Here's how the part is built. I have some questions about the finished solid (model axes, mm). A direction names the side the tool comes from. Round coordinates to 2 decimals unless told otherwise and drop trailing zeros. Write each loop counter-clockwise with the first axis right and the second up, starting at its lowest first coordinate (ties: lowest second). Pieces come first, ordered by that corner, then holes. Notation, with made-up numbers: M 89,-25.5 L 148,-25.5 A22 cw 148,-4.5 Z; hole C 79,63.25 d2. An arc over 180 degrees is marked long. Use one line per item in the form item = value. Start each with the question number.
Q1. I need wall thicknesses on line 1 along Y through (x, z) = (0, 16); line 2 along Y through (x, z) = (0, 3); line 3 along Z through (x, y) = (-8, 13). Which ranges of each line are inside material? Lowest first, please. Write a range as from..to.
Q2. I want a section at D-D on x = -18.5. List the corners of the cut face in (y, z) for me.
Q3. I want a section at C-C on y = 30. List the corners of the cut face in (x, z) for me.
Q4. I want a section at A-A on z = 4. List the corners of the cut face in (x, y) for me.
Q5. I want a section at B-B on x = 4. List the corners of the cut face in (y, z) for me.
Q6. We'd pull the mould along X, two halves only. Please class faces 1 (the face through (28, 0, 60)), 2 (the face through (24.5, 2.65, 55.08)), 3 (the face through (-20.23, 3.62, 9.86)): +X half, -X half, draft (parallel to the pull), parting line (faces both ways), or undercut.
Q7. I'm going to push flat-ended pins straight in: pin 1 Ø13.5 at (x, y) = (2.5, 14.5) entering from +Z; pin 2 Ø5 at (x, y) = (28.5, 8.5) entering from +Z; pin 3 Ø2 at (y, z) = (-1, 15) entering from +X; pin 4 Ø8 at (y, z) = (5.5, 45.5) entering from -X. Where does each tip first touch, or does it pass through?
Q8. For faces 4 (the face through (24.43, -0.61, 44.08)), 5 (the face through (20, 4.15, 58)), 6 (the face through (26.03, 1.64, 57.32)), 7 (the face through (2, 36, 15)), 8 (the face through (20.454, 3.43, 9.86)), which set-ups out of +Z, -Z, +X, -X, +Y, -Y let a thin tool reach every point of the face, with its end or its side?
Autodesk Inventor part; units mm, degrees
ref_plane "YZ Plane" through (0, 0, 0) normal (1, 0, 0) x (0, 1, 0)
ref_plane "XZ Plane" through (0, 0, 0) normal (0, 1, 0) x (-1, 0, 0)
ref_plane "XY Plane" through (0, 0, 0) normal (0, 0, 1) x (1, 0, 0)
sketch "Sketch1" plane through (0, 0, 0) normal (0, 0, 1) x (1, 0, 0)
  circle A0 centre (0, 30) radius 8.45
  circle A1 centre (0, 30) radius 6
  arc A2 (-30, 0) -> (-15.2201, 12.4401) centre (-30, 15) ccw
  arc A3 (15.2201, 12.4401) -> (30, 0) centre (30, 15) ccw
  arc A4 (11.824, 32.0479) -> (-11.824, 32.0479) centre (0, 30) ccw
  line L0 (-11.824, 32.0479) -> (-15.2201, 12.4401)
  line L1 (11.824, 32.0479) -> (15.2201, 12.4401)
  line L2 (30, 0) -> (-30, 0)
  line L3 (-30, 0) -> (-30, -2.5)
  line L4 (-30, -2.5) -> (30, -2.5)
  line L5 (30, -2.5) -> (30, 0)
  point P0 (0, 0)
  point P1 (0, 0)
  point P2 (0, 0)
  dimension "d0" = 16.9
  dimension "d1" = 12
  dimension "d2" = 30
  dimension "d3" = 12
  dimension "d4" = 15
  dimension "d5" = 60
  dimension "d6" = 2.5
extrude "Extrusion1" add sketch "Sketch1" along normal blind 20 contours A2 L0 A4 L1 A3 L2
extrude "Extrusion2" add sketch "Sketch1" along normal blind 15 contours A0
extrude "Extrusion3" add sketch "Sketch1" along normal blind 20 contours L2 L5 L4 L3
ref_plane "Work Plane1" through (-30, -2.5, 0) normal (0, -1, 0) x (1, 0, 0)
sketch "Sketch2" plane through (-30, -2.5, 0) normal (0, -1, 0) x (1, 0, 0)
  line L0 (21.55, 20) -> (38.45, 20)
  line L1 (30, 20) -> (30, 60) construction
  line L2 (60, 0) -> (60, 20) construction
  line L3 (30, 20) -> (52.9431, 52.7661) construction
  line L4 (47.9062, 63.0072) -> (64.2892, 51.5357)
  line L5 (64.2892, 51.5357) -> (61.1346, 47.0303)
  line L6 (61.1346, 47.0303) -> (44.7515, 58.5018) construction
  line L7 (44.7515, 58.5018) -> (47.9062, 63.0072)
  line L8 (44.7515, 58.5018) -> (17.7923, 20)
  line L9 (41.824, 20) -> (18.176, 20)
  line L10 (61.1346, 47.0303) -> (42.2077, 20)
  line L11 (0, 20) -> (60, 20)
  point P0 (30, 0)
  dimension "d14" = 35
  dimension "d16" = 5.5
  dimension "d17" = 20
  dimension "d26" = 40
extrude "Extrusion6" add sketch "Sketch2" against normal blind 2.5
sketch "Sketch4" plane through (34.2892, -2.5, 51.5357) normal (0.5735764, 0, 0.819152) x (0.819152, 0, -0.5735764)
  line L0 (-23.103, 0) -> (-34.5746, 0)
  circle A0 centre (-10, 10.5) radius 7.3 construction
  circle A1 centre (-10, 10.5) radius 5.35
  line L1 (-16.2022, 2.5) -> (-3.7978, 2.5)
  line L2 (-3.7978, 2.5) -> (-3.7978, 6.65)
  line L3 (-3.7978, 6.65) -> (-16.2022, 6.65)
  line L4 (-16.2022, 6.65) -> (-16.2022, 2.5)
  line L5 (-20, 2.5) -> (0, 2.5)
  line L6 (-16.2022, 2.5) -> (-16.2022, 0)
  line L7 (-3.7978, 2.5) -> (-3.7978, 0)
  line L8 (-23.103, 0) -> (26.0461, 0)
  line L9 (0, 0) -> (-20, 0)
  line L10 (0, 0) -> (0, 2.5)
  line L11 (-20, 2.5) -> (0, 2.5)
  line L12 (-20, 0) -> (-20, 2.5)
  point P0 (1.4715, 2.5)
  point P1 (-10, 2.5)
  point P2 (-6.2852, 6.65)
  point P3 (-13.7148, 6.65)
  point P4 (0, 0)
  point P5 (0, 2.5)
  point P6 (-20, 2.5)
  point P7 (-20, 0)
  point P8 (-16.2022, 2.5)
  dimension "d29" = 14.6
  dimension "d30" = 10.7
  dimension "d31" = 1.5
  dimension "d32" = 8
extrude "Extrusion7" add sketch "Sketch4" against normal blind 5.5 contours A1 L3 L2 L1 L4
extrude "Extrusion8" cut sketch "Sketch4" against normal up to surface contours L6 L8 L12 L5 | L5 L10 L8 L7 surface through (0, 21, 20) normal (0, 0, 1)
extrude "Extrusion9" add sketch "Sketch4" along normal blind 7.5 contours L1 L7 L8 L6
properties part number "Support 1 - V2"
Reported:
q1.line_1 = -2.5..21.55, 38.45..42
q1.line_2 = -2.5..24, 36..42
q1.line_3 = 0..20
q2.outline = M -2.5,0 L 5.37,0 L 5.37,20 L -2.5,20 Z
q3.outline = M -12.18,0 L -6,0 L -6,15 L -8.45,15 L -8.45,20 L -12.18,20 Z; M 6,0 L 12.18,0 L 12.18,20 L 8.45,20 L 8.45,15 L 6,15 Z
q4.outline = M -30,-2.5 L 30,-2.5 L 30,0 A15 cw 15.22,12.44 L 11.82,32.05 A12 ccw -11.82,32.05 L -15.22,12.44 A15 cw -30,0 Z; hole C 0,30 d12
q5.outline = M -2.5,0 L 25.53,0 L 25.53,15 L 22.56,15 L 22.56,20 L 0,20 L 0,36.53 L -2.5,36.53 Z; M 34.47,0 L 41.31,0 L 41.31,20 L 37.44,20 L 37.44,15 L 34.47,15 Z
q6.face_1 = draft
q6.face_2 = undercut
q6.face_3 = -X half
q7.pin_1 = 20
q7.pin_2 = through
q7.pin_3 = 30
q7.pin_4 = 27.94
q8.face_4 = +X, +Y, -Y
q8.face_5 = +Z, +X, -X, +Y
q8.face_6 = +Z, +X, +Y
q8.face_7 = +Z
q8.face_8 = -Z, +X, +Y
